Autodesk Inventor part; units mm, degrees
ref_plane "YZ Plane" through (0, 0, 0) normal (1, 0, 0) x (0, 1, 0)
ref_plane "XZ Plane" through (0, 0, 0) normal (0, 1, 0) x (-1, 0, 0)
ref_plane "XY Plane" through (0, 0, 0) normal (0, 0, 1) x (1, 0, 0)
sketch "Sketch1" plane through (0, 0, 0) normal (0, 0, 1) x (1, 0, 0)
  circle A0 centre (0, 0) radius 14
  dimension "d0" = 28
extrude "Extrusion1" add sketch "Sketch1" along normal blind 19
sketch "Sketch2" plane through (0, 0, 19) normal (0, 0, 1) x (1, 0, 0)
  line L0 (10, 7.5) -> (16, 7.5)
  line L1 (16, 7.5) -> (16, -7.5)
  line L2 (16, -7.5) -> (10, -7.5)
  line L3 (10, -7.5) -> (10, 7.5)
  point P0 (0, 0)
  dimension "d3" = 15
  dimension "d4" = 10
  dimension "d5" = 16
  dimension "d6" = 7.5
extrude "Extrusion2" add sketch "Sketch2" against normal blind 16.5
fillet "Fillet1" radius 1 2 edges at (16, 7.5, 10.75) (16, -7.5, 10.75)
sketch "Sketch3" plane through (0, 0, 19) normal (0, 0, 1) x (1, 0, 0)
  circle A0 centre (-8, 0) radius 4.5
  arc A1 (11.8216, 7.5) -> (11.8216, -7.5) centre (0, 0) ccw
  dimension "d10" = 9
  dimension "d11" = 0
  dimension "d12" = 8
extrude "Extrusion3" add sketch "Sketch3" along normal blind 2
sketch "Sketch4" plane through (-8, 0, 21) normal (0, 0, 1) x (1, 0, 0)
  circle A0 centre (0, 0) radius 2.5
  point P0 (8, 0)
  dimension "d15" = 5
extrude "Extrusion4" add sketch "Sketch4" along normal blind 8
sketch "Sketch5" plane through (-8, 0, 29) normal (0, 0, 1) x (1, 0, 0)
  circle A0 centre (0, 0) radius 2.5
  circle A1 centre (0, 0) radius 2.5
  line L0 (-3.3103, 1.5) -> (3.6339, 1.5)
  line L1 (3.6339, 1.5) -> (3.6339, -1.5)
  line L2 (3.6339, -1.5) -> (-3.3103, -1.5)
  line L3 (-3.3103, -1.5) -> (-3.3103, 1.5)
  point P0 (8, 0)
  point P1 (2, -1.5)
  point P2 (-2, -1.5)
  point P3 (-2, 1.5)
  point P4 (2, 1.5)
  dimension "d18" = 3
  dimension "d19" = 1.5
extrude "Extrusion5" cut sketch "Sketch5" against normal blind 6 contours L0 A0 | A0 L2
sketch "Sketch6" plane through (16, -6.5, 19) normal (1, 0, 0) x (0, 0, -1)
  line L0 (2, 10.5) -> (3, 10.5)
  line L1 (3, 10.5) -> (3, 2.5)
  line L2 (3, 2.5) -> (2, 2.5)
  line L3 (2, 2.5) -> (2, 10.5)
  line L4 (0, 0) -> (0, 13)
  line L5 (16.5, 14) -> (0, 14)
  line L6 (0, -1) -> (16.5, -1)
  point P0 (19, 6.5)
  dimension "d22" = 2
  dimension "d23" = 1
  dimension "d24" = 3.5
  dimension "d25" = 3.5
extrude "Extrusion6" add sketch "Sketch6" along normal blind 5
sketch "Sketch7" plane through (0, 0, 19) normal (0, 0, 1) x (1, 0, 0)
  line L0 (-3.5, 12) -> (3.5, 12)
  line L1 (3.5, 12) -> (3.5, 21)
  line L2 (3.5, 21) -> (-3.5, 21)
  line L3 (-3.5, 21) -> (-3.5, 12)
  arc A0 (11.8216, 7.5) -> (11.8216, -7.5) centre (0, 0) ccw
  line L4 (-3.5, -12) -> (3.5, -12)
  line L5 (3.5, -12) -> (3.5, -21)
  line L6 (3.5, -21) -> (-3.5, -21)
  line L7 (-3.5, -21) -> (-3.5, -12)
  point P0 (0, 14)
  point P1 (0, -14)
  point P2 (3.5, -13.5554)
  point P3 (-3.5, -13.5554)
  point P4 (-3.5, 13.5554)
  point P5 (3.5, 13.5554)
  dimension "d28" = 7
  dimension "d29" = 7
  dimension "d30" = 3.5
  dimension "d31" = 2
  dimension "d32" = 7
  dimension "d33" = 7
  dimension "d34" = 2
  dimension "d35" = 3.5
extrude "Extrusion7" add sketch "Sketch7" against normal blind 0.5 contours A0 L5 L6 L7 | L3 L2 L1 A0
fillet "Fillet2" radius 3.5 4 edges at (-3.5, 21, 18.75) (3.5, 21, 18.75) (-3.5, -21, 18.75) (3.5, -21, 18.75)
sketch "Sketch8" plane through (0, 0, 19) normal (0, 0, 1) x (1, 0, 0)
  arc A0 (3.5, 17.5) -> (-3.5, 17.5) centre (0, 17.5) ccw
  arc A1 (-3.5, -17.5) -> (3.5, -17.5) centre (0, -17.5) ccw
  point P0 (0, 0)
  dimension "d39" = 0
hole "Hole1" at (0, 17.5, 19) at (0, -17.5, 19) direction (0, 0, -1) diameter 4 depth 1 tip angle 118
properties part number "stepper-motor"
Verification items for the finished model (mm, model axes). A direction names the side the tool comes from. Coordinates: 2 decimals unless noted, no trailing zeros. Order: outer loops, then holes, each group sorted by start corner. A loop starts at its lowest first (then second) coordinate and runs counter-clockwise, first axis right, second up. Notation, with made-up numbers: (50.5, -16) - (90.5, -16) arc R29 ccw to (90.5, 7) - close; hole circle Ø5 at (-29, 32.5). An arc over 180 degrees is marked (long way). Return JSON: item names as keys, results as strings.
(1) Mould release check, pull along Y, two halves, no side actions. Record for faces 4 (the flat face through (18.5, 4, 16.5)), 5 (the cylindrical face through (-3.708, -1.352, 19.986)), 6 (the cylindrical face through (1.2, -15.9, 18.7)), 7 (the flat face through (18, 0, 16)): pulls with the +Y half, pulls with the -Y half, needs draft (parallel to the pull), parting line crosses it, or undercut.
Filled sheet:
{"face 4": "pulls with the +Y half", "face 5": "parting line crosses it", "face 6": "undercut", "face 7": "needs draft"}
(2) Section check C-C, the plane z = 5.5. Record the cut outline in (x, y), and give its area (3 significant figures).
Filled sheet:
{"outline": "(11.82, -7.5) - (15, -7.5) arc R1 ccw to (16, -6.5) - (16, 6.5) arc R1 ccw to (15, 7.5) - (11.82, 7.5) arc R14 ccw (long way) to start", "area": "656 mm^2"}
(3) Section check D-D, the plane x = -8. Record the cut outline in (y, z), and give its area (3 significant figures).
Filled sheet:
{"outline": "(-11.49, 0) - (11.49, 0) - (11.49, 19) - (4.5, 19) - (4.5, 21) - (2.5, 21) - (2.5, 23) - (1.5, 23) - (1.5, 29) - (-1.5, 29) - (-1.5, 23) - (-2.5, 23) - (-2.5, 21) - (-4.5, 21) - (-4.5, 19) - (-11.49, 19) - close", "area": "483 mm^2"}
(4) Thickness scan on line 1 along Y through (x, z) = (0, 18.7); line 2 along Y through (x, z) = (13.5, 5.75); line 3 along Z through (x, y) = (-12, -0.5). Record the ranges inside material, lowest first.
Filled sheet:
{"line 1": "y = -21 to -19.5, -15.5 to 15.5, 19.5 to 21", "line 2": "y = -7.5 to 7.5", "line 3": "z = 0 to 21"}
(5) Go/stop test with flat-tipped pins: pin 1 (0.6 mm diameter, centred on y = -16, z = 18.5, fed in from -X); pin 2 (0.8 mm diameter, centred on x = -8.5, y = -2, fed in from +Z); pin 3 (1 mm diameter, centred on x = 12.5, z = 13.5, fed in from +Y); pin 4 (3 mm diameter, centred on x = 0, y = 17.5, fed in from -Z). Record where each tip stops, or that it passes through.
Filled sheet:
{"pin 1": "stops at x = -3.5", "pin 2": "stops at z = 23", "pin 3": "stops at y = 7.5", "pin 4": "passes through"}
(6) Section check B-B, the plane y = 17. Record the cut outline in (x, z).
Filled sheet:
{"outline": "(-3.5, 18.5) - (-1.94, 18.5) - (-1.94, 19) - (-3.5, 19) - close; (1.94, 18.5) - (3.5, 18.5) - (3.5, 19) - (1.94, 19) - close"}
(7) Access from +Z, -Z, +X, -X, +Y, -Y to the whole of each face (thin tool, end or side, straight path). Record for faces 1 (the flat face through (13, 7.5, 11)), 2 (the flat face through (-8, -1.5, 26)), 3 (the cylindrical face through (-13.986, -0.616, 9.367)).
Filled sheet:
{"face 1": "+Z, -Z, +X, +Y", "face 2": "+Z, +X, -X, -Y", "face 3": "-Z"}
(8) Section check A-A, the plane y = 0. Record the cut outline in (x, z), and give its area (3 significant figures).
Filled sheet:
{"outline": "(-14, 0) - (14, 0) - (14, 2.5) - (16, 2.5) - (16, 16) - (21, 16) - (21, 17) - (16, 17) - (16, 19) - (-3.5, 19) - (-3.5, 21) - (-5.5, 21) - (-5.5, 29) - (-10.5, 29) - (-10.5, 21) - (-12.5, 21) - (-12.5, 19) - (-14, 19) - close", "area": "628 mm^2"}
